Can you work these out from the model? Positions are in its coordinate system, mm. Face numbers are marked on the shaded views. Give positions to 0.01 mm unless a question says otherwise; leave off trailing zeros. Loops run counter-clockwise (first coordinate to the right, second up) from the corner with the lowest first, then second, coordinate; pieces in that order, holes last.
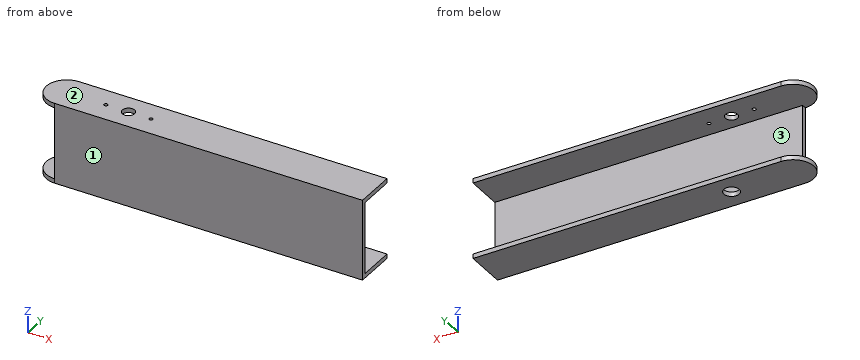
from build123d import *

# Parameters (mm, degrees)
BOSS_EXTRUDE1_DEPTH = 2.7686
SKETCH3_R           = 3.81
SKETCH3_R_2         = 1.1303
CUT_EXTRUDE1_DEPTH  = 3.7686
BOSS_EXTRUDE2_START = -2.7686
SKETCH5_W           = 190.5
SKETCH5_H           = 2.7686
BOSS_EXTRUDE2_DEPTH = 44.45
BOSS_EXTRUDE3_DEPTH = 2.7686
SKETCH7_R           = 4.7625
CUT_EXTRUDE2_DEPTH  = 2.7686


with BuildPart() as part:
    # Sketch1 → Boss-Extrude1 (new body)
    with BuildSketch(Plane.XY):
        with BuildLine():
            Line((0, 0), (190.499997766, 0))
            Line((190.499997766, 0), (190.499997766, 25.4))
            Line((190.499997766, 25.4), (-4.468e-06, 25.4))
            ThreePointArc((-4.468e-06, 25.4), (-12.700002234, 12.699997766), (0, 0))
        make_face()
    extrude(amount=BOSS_EXTRUDE1_DEPTH)

    # Sketch3 → Cut-Extrude1 (cut, through all)
    with BuildSketch(Plane.XY.offset(2.7686)):
        with Locations((38.099997766, 12.7)):
            Circle(SKETCH3_R)
        with Locations((24.129997766, 12.7)):
            Circle(SKETCH3_R_2)
        with Locations((52.069997766, 12.7)):
            Circle(SKETCH3_R_2)
    extrude(amount=-CUT_EXTRUDE1_DEPTH, mode=Mode.SUBTRACT)

    # Sketch5 → Boss-Extrude2 (add)
    with BuildSketch(Plane.XY.offset(2.7686).offset(BOSS_EXTRUDE2_START)):
        with Locations((95.249997766, 1.3843)):
            Rectangle(SKETCH5_W, SKETCH5_H)
    extrude(amount=-BOSS_EXTRUDE2_DEPTH)

    # Sketch6 → Boss-Extrude3 (add)
    with BuildSketch(Plane(origin=(0, 0, -44.45), x_dir=(-1, 0, 0), z_dir=(0, 0, -1))):
        with BuildLine():
            Line((4.468e-06, 25.4), (-190.499997766, 25.4))
            Line((-190.499997766, 25.4), (-190.499997766, 12.7))
            Line((-190.499997766, 12.7), (-190.499997766, 0))
            Line((-190.499997766, 0), (0, 0))
            ThreePointArc((0, 0), (12.700002234, 12.699997766), (4.468e-06, 25.4))
        make_face()
    extrude(amount=BOSS_EXTRUDE3_DEPTH)

    # Sketch7 → Cut-Extrude2 (cut)
    with BuildSketch(Plane(origin=(0, 0, -47.2186), x_dir=(-1, 0, 0), z_dir=(0, 0, -1))):
        with Locations((-38.099997766, 12.7)):
            Circle(SKETCH7_R)
    extrude(amount=-CUT_EXTRUDE2_DEPTH, mode=Mode.SUBTRACT)


solid = part.part
(1) Will these pins go through, and if not, where does the flat tip stop? P1, Ø5, axis at y = 4, z = -5, coming from the -X side; P2, Ø3, axis at x = 147.5, z = -10, coming from the +Y side.
Returned:
P1: stops at x = 0
P2: stops at y = 2.77
(2) Suppose I cut it at B-B on z = -15. List the corners of the cut face in (x, y) for me.
Returned:
outline: (0, 0) - (190.5, 0) - (190.5, 2.77) - (0, 2.77) - close
(3) Suppose I cut it at A-A on x = 66.5. List the corners of the cut face in (y, z) for me.
Returned:
outline: (0, -47.22) - (25.4, -47.22) - (25.4, -44.45) - (2.77, -44.45) - (2.77, 0) - (25.4, 0) - (25.4, 2.77) - (0, 2.77) - close
(4) Thinking about a two-plate mould opening in Z: for the marked faces 1, 2 and 3, which applies, pulls with the +Z half, pulls with the -Z half, needs draft (parallel to the pull), parting line crosses it, or undercut?
Returned:
face 1: needs draft
face 2: pulls with the +Z half
face 3: undercut
(5) Please list where these lines run through material, in increasing order: probe 1 along Z at (x, y) = (49, 18.5); probe 2 along Y at (x, z) = (18, -15.5).
Returned:
probe 1: z = -47.22 to -44.45, 0 to 2.77
probe 2: y = 0 to 2.77
